Can you work these out from the model? Positions are in its coordinate system, mm. Give positions to 0.01 mm unless a question says otherwise; leave off trailing zeros. Order: outer loops, then holes, each group sorted by start corner. A loop starts at its lowest first (then second) coordinate and runs counter-clockwise, first axis right, second up.
Item 1: If I drill on line 1 along Y through (x, z) = (27, 23); line 2 along Y through (x, z) = (36, 11.25); line 3 along X through (y, z) = (11.5, 18.75), over which ranges is the centre line in solid material (lowest first)?
Item 2: I'm going to push a flat-ended pin straight in: pin 1 Ø2 at (y, z) = (22.5, 14.5) entering from -X. Where does the tip first touch, or does it pass through?
Item 3: I want a section at A-A, the plane y = 9.5. Write out the boundary of the cut face in (x, z).
Item 4: If we mould it in two halves opening along Z, with no side actions, what happens to faces 1 (the flat face through (20, 27, 25.4)), 2 (the flat face through (48.499, 33, 6)), 3 (the cylindrical face through (2.732, 26.768, 9.351))? For each: +Z half, -Z half, draft (parallel to the pull), parting line (faces both ways), or undercut.
```python
from build123d import *

# Parameters (mm, degrees)
F0_W        = 48.4990663826
F0_H        = 54.2960166931
F1_DEPTH    = 25.4
F4_T1_DEPTH = 73.8990663826
F4_T3_DEPTH = 55.000743558
F4_T5_DEPTH = 60.9725440939
F4_T7_DEPTH = 82.7166388813


# Not quite as in the source:
# - a fillet or chamfer that OpenCascade refuses, or shapes differently, is made with other operations: its cross-section is extruded or revolved along the edge and cut away or added


with BuildPart() as f1:
    # F0 (on Top) → F1 (new body)
    with BuildSketch(Plane.XY):
        with Locations((24.2495331913, 27.1480083466)):
            Rectangle(F0_W, F0_H)
    extrude(amount=F1_DEPTH)

    # F2 (on face) → F3 (revolve, intersect)
    with BuildSketch(Plane.XY.offset(25.4)):
        with BuildLine():
            ThreePointArc((48.4990663826, 20.710743558), (25.7133262446, 24.1621080786), (48.4990663826, 27.6134725992))
            Line((48.4990663826, 27.6134725992), (48.4990663826, 54.2960166931))
            Line((48.4990663826, 54.2960166931), (0, 54.2960166931))
            Line((0, 54.2960166931), (0, 0))
            Line((0, 0), (48.4990663826, 0))
            Line((48.4990663826, 0), (48.4990663826, 20.710743558))
        make_face()
    revolve(axis=Axis((48.4990663826, 27.1480083466, 25.4), (0, 1, 0)), mode=Mode.INTERSECT)

    # F4: fillet of radius 5.08 on 5 edges, made by hand

    # F4_s2 → F4_t1 (cut)
    with BuildSketch(Plane.YZ.offset(-12.7)):
        with BuildLine():
            ThreePointArc((5.08, 25.4), (1.4878975516, 23.9121024484), (0, 20.32))
            Line((0, 20.32), (0, 25.4))
            Line((0, 25.4), (5.08, 25.4))
        make_face()
        with BuildLine():
            ThreePointArc((49.2160166931, 25.4), (52.8081191415, 23.9121024484), (54.2960166931, 20.32))
            Line((54.2960166931, 20.32), (54.2960166931, 25.4))
            Line((54.2960166931, 25.4), (49.2160166931, 25.4))
        make_face()
    extrude(amount=F4_T1_DEPTH, mode=Mode.SUBTRACT)

    # F4_s4 → F4_t3 (cut)
    with BuildSketch(Plane.XZ.offset(-42.300743558)):
        with BuildLine():
            ThreePointArc((43.4190663826, 25.4), (47.0111688311, 23.9121024484), (48.4990663826, 20.32))
            Line((48.4990663826, 20.32), (48.4990663826, 25.4))
            Line((48.4990663826, 25.4), (43.4190663826, 25.4))
        make_face()
    extrude(amount=F4_T3_DEPTH, mode=Mode.SUBTRACT)

    # F4_s6 → F4_t5 (cut)
    with BuildSketch(Plane.XZ.offset(-66.9960166931)):
        with BuildLine():
            ThreePointArc((43.4190663826, 25.4), (47.0111688311, 23.9121024484), (48.4990663826, 20.32))
            Line((48.4990663826, 20.32), (48.4990663826, 25.4))
            Line((48.4990663826, 25.4), (43.4190663826, 25.4))
        make_face()
    extrude(amount=F4_T5_DEPTH, mode=Mode.SUBTRACT)

    # F4_s8 → F4_t7 (cut)
    with BuildSketch(Plane.XZ.offset(-68.5063277872)):
        with BuildLine():
            ThreePointArc((5.3782022269, 25.4), (1.5817742667, 23.6954310455), (0.3330916761, 19.7256435997))
            ThreePointArc((0.3330916761, 19.7256435997), (0.0833445319, 22.5579377812), (0, 25.4))
            Line((0, 25.4), (5.3782022269, 25.4))
        make_face()
    extrude(amount=F4_T7_DEPTH, mode=Mode.SUBTRACT)


solid = f1.part
```
Results list:
1. line 1: y = 0.76 to 19.11, 29.22 to 53.53
1. line 2: y = 0 to 15.46, 32.87 to 54.3
1. line 3: x = 0.46 to 48.5
2. pin 1: stops at x = 1.02
3. outline: (0.33, 19.73) arc R48.5 ccw to (7.18, 0) - (48.5, 0) - (48.5, 20.32) arc R5.08 ccw to (43.42, 25.4) - (5.38, 25.4) arc R5.08 ccw to start
4. face 1: +Z half
4. face 2: draft
4. face 3: -Z half
